Source: CAD feature listing. Evaluate the final solid. Frame: model axes, mm. Face numbers are marked on the shaded views. A direction names the side the tool comes from. Round coordinates to 2 decimals unless told otherwise and drop trailing zeros. Loops run counter-clockwise (first coordinate to the right, second up) from the corner with the lowest first, then second, coordinate; pieces in that order, holes last. Notation, with made-up numbers: M 70,36 L 90,36 A27 cw 90,69 Z; hole C 28,36.25 d9. An arc over 180 degrees is marked long. Answer as a JSON object with one key per item and string values.
from build123d import *

# Parameters (mm, degrees)
SKETCH_1_W          = 140
SKETCH_1_H          = 100
EXTRUDE_1_DEPTH     = 4
SKETCH_9_R          = 2.75
CUT_EXTRUDE_3_DEPTH = 8
CHAMFER_2_SIZE      = 2
SKETCH_11_W         = 40
SKETCH_11_H         = 50
CUT_EXTRUDE_5_DEPTH = 5
SKETCH_12_W         = 10
SKETCH_12_H         = 15
EXTRUDE_2_DEPTH     = 14
SKETCH_13_W         = 60
SKETCH_13_H         = 15
EXTRUDE_3_DEPTH     = 14
EXTRUDE_4_DEPTH     = 20
EXTRUDE_5_DEPTH     = 20
SKETCH_16_R         = 6.75
CUT_EXTRUDE_6_DEPTH = 20
EXTRUDE_6_DEPTH     = 10
SKETCH_18_R         = 2.75
CUT_EXTRUDE_7_DEPTH = 96.268042911
SKETCH_19_R         = 2.75
CUT_EXTRUDE_8_DEPTH = 100
CHAMFER_3_SIZE      = 0.5
EXTRUDE_7_DEPTH     = 20
EXTRUDE_8_DEPTH     = 20
FILLET_1_R          = 5


with BuildPart() as part:
    # 草图1 → 凸台-拉伸1 (new body)
    with BuildSketch(Plane(origin=(0, 0, 0), x_dir=(0, 0, -1), z_dir=(1, 0, 0))):
        with Locations((0, -10)):
            Rectangle(SKETCH_1_W, SKETCH_1_H)
    extrude(amount=EXTRUDE_1_DEPTH)

    # 草图9 → 切除-拉伸3 (cut)
    with BuildSketch(Plane(origin=(4, 0, 0), x_dir=(0, 0, -1), z_dir=(1, 0, 0))):
        with Locations((-60, 20)):
            Circle(SKETCH_9_R)
        with Locations((60, 20)):
            Circle(SKETCH_9_R)
        with Locations((-45, -40)):
            Circle(SKETCH_9_R)
        with Locations((45, -40)):
            Circle(SKETCH_9_R)
    extrude(amount=-CUT_EXTRUDE_3_DEPTH, mode=Mode.SUBTRACT)

    # 倒角2
    chamfer_2_edges = [part.edges().sort_by_distance(p)[0] for p in [
        (2, 40, 70),
        (2, 40, -70),
        (2, -60, -70),
        (2, -60, 70),
    ]]
    chamfer(chamfer_2_edges, length=CHAMFER_2_SIZE)

    # 草图11 → 切除-拉伸5 (cut)
    with BuildSketch(Plane(origin=(4, 0, 0), x_dir=(0, 0, -1), z_dir=(1, 0, 0))):
        with Locations((0, 15)):
            Rectangle(SKETCH_11_W, SKETCH_11_H)
    extrude(amount=-CUT_EXTRUDE_5_DEPTH, mode=Mode.SUBTRACT)

    # 草图12 → 凸台-拉伸2 (add)
    with BuildSketch(Plane(origin=(4, 0, 0), x_dir=(0, 0, -1), z_dir=(1, 0, 0))):
        with Locations((-25, 32.5)):
            Rectangle(SKETCH_12_W, SKETCH_12_H)
        with Locations((25, 32.5)):
            Rectangle(SKETCH_12_W, SKETCH_12_H)
    extrude(amount=EXTRUDE_2_DEPTH)

    # 草图13 → 凸台-拉伸3 (add)
    with BuildSketch(Plane(origin=(18, 0, 0), x_dir=(0, 0, -1), z_dir=(1, 0, 0))):
        with Locations((0, 32.5)):
            Rectangle(SKETCH_13_W, SKETCH_13_H)
    extrude(amount=EXTRUDE_3_DEPTH)

    # 草图14 → 凸台-拉伸4 (add)
    with BuildSketch(Plane.XY.offset(30)):
        Polygon((4, 40), (4, -30), (32, 25), (32, 40), align=None)
    extrude(amount=EXTRUDE_4_DEPTH)

    # 草图15 → 凸台-拉伸5 (add)
    with BuildSketch(Plane(origin=(0, 0, -30), x_dir=(-1, 0, 0), z_dir=(0, 0, -1))):
        Polygon((-4, 40), (-32, 40), (-32, 25), (-4, -30), align=None)
    extrude(amount=EXTRUDE_5_DEPTH)

    # 草图16 → 切除-拉伸6 (cut)
    with BuildSketch(Plane(origin=(0, 40, 0), x_dir=(1, 0, 0), z_dir=(0, 1, 0))):
        with Locations((18, 0)):
            Circle(SKETCH_16_R)
    extrude(amount=-CUT_EXTRUDE_6_DEPTH, mode=Mode.SUBTRACT)

    # 草图17 → 凸台-拉伸6 (add)
    with BuildSketch(Plane(origin=(32, 0, 0), x_dir=(0, 0, -1), z_dir=(1, 0, 0))):
        Polygon((50, 40), (-50, 40), (-50, 25), (-30, 25), (30, 25), (50, 25), align=None)
    extrude(amount=EXTRUDE_6_DEPTH)

    # 草图18 → 切除-拉伸7 (cut, through all)
    with BuildSketch(Plane.ZY.offset(-18)):
        with Locations((14, 32.5)):
            Circle(SKETCH_18_R)
        with Locations((-14, 32.5)):
            Circle(SKETCH_18_R)
    extrude(amount=-CUT_EXTRUDE_7_DEPTH, mode=Mode.SUBTRACT)

    # 草图19 → 切除-拉伸8 (cut)
    with BuildSketch(Plane(origin=(42, 0, 0), x_dir=(0, 0, -1), z_dir=(1, 0, 0))):
        with Locations((0, 32.5)):
            Circle(SKETCH_19_R)
    extrude(amount=-CUT_EXTRUDE_8_DEPTH, mode=Mode.SUBTRACT)

    # 倒角3
    chamfer_3_edges = [part.edges().sort_by_distance(p)[0] for p in [
        (4, 20, 62.75),
        (4, -40, -42.25),
        (4, -40, 47.75),
        (4, 20, -57.25),
    ]]
    chamfer(chamfer_3_edges, length=CHAMFER_3_SIZE)

    # 草图20 → 凸台-拉伸7 (add)
    with BuildSketch(Plane.XY.offset(50)):
        Polygon((42, 25), (4, -30), (32, 25), align=None)
    extrude(amount=-EXTRUDE_7_DEPTH)

    # 草图21 → 凸台-拉伸8 (add)
    with BuildSketch(Plane(origin=(0, 0, -50), x_dir=(-1, 0, 0), z_dir=(0, 0, -1))):
        Polygon((-42, 25), (-4, -30), (-32, 25), align=None)
    extrude(amount=-EXTRUDE_8_DEPTH)

    # 圆角1
    fillet_1_edges = [part.edges().sort_by_distance(p)[0] for p in [
        (42, 32.5, -50),
        (42, 32.5, 50),
    ]]
    fillet(fillet_1_edges, radius=FILLET_1_R)


solid = part.part
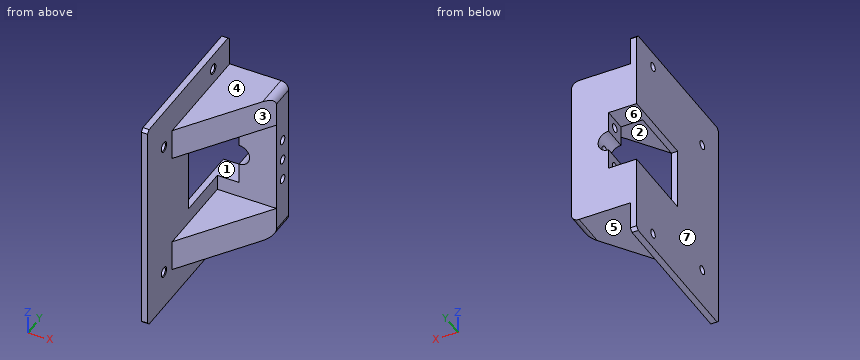
Item 1: Line query: probe 1 along Z at (x, y) = (10, 0.5); probe 2 along Z at (x, y) = (25.5, 33); probe 3 along Z at (x, y) = (20, 34). Output: solid intervals per line, ascending. Write a range as from..to.
Answer sheet:
{"probe 1": "z = -50..-30, 30..50", "probe 2": "z = -50..-16.7, -11.3..-2.7, 2.7..11.3, 16.7..50", "probe 3": "z = -50..-16.3, -11.7..-6.45, 6.45..11.7, 16.3..50"}
Item 2: Section A-A on z = -60. Return the cut outline in (x, y).
Answer sheet:
{"outline": "M 0,-60 L 4,-60 L 4,16.75 L 3.5,17.25 L 0,17.25 Z; M 0,22.75 L 3.5,22.75 L 4,23.25 L 4,40 L 0,40 Z"}
Item 3: Access query for the marked faces 1, 2, 3 and 4. Directions: +Z, -Z, +X, -X, +Y, -Y. A direction counts if a zero-diameter tool reaches every point of the face in a straight line with its end or side. Return the directions, or none.
Answer sheet:
{"face 1": "-X, +Y", "face 2": "+X, -Y", "face 3": "+Z, -Z, +X, -Y", "face 4": "+Z, +X, +Y, -Y"}
Item 4: Section D-D on x = 13. Return the cut outline in (y, z).
Answer sheet:
{"outline": "M -16.97,-50 L 40,-50 L 40,-20 L 25,-20 L 25,-30 L -16.97,-30 Z; M -16.97,30 L 25,30 L 25,20 L 40,20 L 40,50 L -16.97,50 Z"}
Item 5: Section C-C on z = -14. Return the cut outline in (x, y), then the cut area to 3 significant figures.
Answer sheet:
{"outline": "M 0,-60 L 4,-60 L 4,-10 L 0,-10 Z; M 18,25 L 42,25 L 42,29.75 L 18,29.75 Z; M 18,35.25 L 42,35.25 L 42,40 L 18,40 Z", "area": "428 mm²"}
Item 6: Contact query for flat-ended pins moving along their axis: pin 1 Ø10 at (x, y) = (29.5, 8.5) entering from +Z; pin 2 Ø10 at (x, z) = (28.5, 11.5) entering from -Y; pin 3 Ø8 at (x, z) = (12.5, 43) entering from -Y. Output: stop coordinate, or through.
Answer sheet:
{"pin 1": "stops at z = 50", "pin 2": "stops at y = 25", "pin 3": "stops at y = -23.49"}
Item 7: Section B-B on y = 32.5. Return the cut outline in (x, z).
Answer sheet:
{"outline": "M 0,-70 L 4,-70 L 4,-50 L 37,-50 A5 ccw 42,-45 L 42,-16.75 L 18,-16.75 L 18,-20 L 0,-20 Z; M 0,20 L 18,20 L 18,16.75 L 42,16.75 L 42,45 A5 ccw 37,50 L 4,50 L 4,70 L 0,70 Z; M 18,-11.25 L 42,-11.25 L 42,-2.75 L 24.16,-2.75 A6.75 cw 18,-6.75 Z; M 18,6.75 A6.75 cw 24.16,2.75 L 42,2.75 L 42,11.25 L 18,11.25 Z"}
Item 8: Pull-direction query (Z, two-part tool) for the marked faces 5, 6 and 7; classes: pulls with the +Z half, pulls with the -Z half, needs draft (parallel to the pull), parting line crosses it, or undercut.
Answer sheet:
{"face 5": "pulls with the -Z half", "face 6": "undercut", "face 7": "needs draft"}
